Autodesk Inventor part; units mm, degrees
ref_plane "YZ Plane" through (0, 0, 0) normal (1, 0, 0) x (0, 1, 0)
ref_plane "XZ Plane" through (0, 0, 0) normal (0, 1, 0) x (-1, 0, 0)
ref_plane "XY Plane" through (0, 0, 0) normal (0, 0, 1) x (1, 0, 0)
sketch "Sketch1" plane through (0, 0, 0) normal (0, 0, 1) x (1, 0, 0)
  line L0 (-40, 12.5) -> (40, 12.5)
  line L1 (40, 12.5) -> (40, -12.5)
  line L2 (40, -12.5) -> (-40, -12.5)
  line L3 (-40, -12.5) -> (-40, 12.5)
  line L4 (-58.4065, 0) -> (96.114, 0) construction
  line L5 (0, 47.121) -> (0, -49.5625) construction
  line L6 (20, 12.5) -> (20, -12.5)
  line L7 (20, 12.5) -> (40, 5.2206)
  line L8 (20, -12.5) -> (40, -5.2206)
  point P0 (0, 0)
  point P1 (0, 12.5)
  point P2 (40, 0)
  dimension "d0" = 80
  dimension "d1" = 25
  dimension "d11" = 20
  dimension "d16" = 70
  dimension "d17" = 70
extrude "Extrusion4" add sketch "Sketch1" along normal blind 0.2 contours L0 L6 L2 L3 | L7 L1 L8 L6
extrude "Extrusion5" add sketch "Sketch1" along normal blind 0.4 contours L7 L1 L8 L6
equation "\"d18\" = material"
equation "\"d20\" = 2 * material"
properties part number "BandBack"
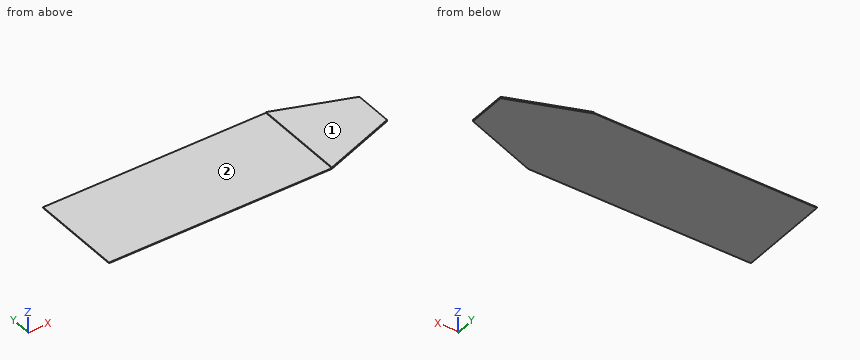
Part model, mm, in its own coordinate system. Face numbers are marked on the shaded views. A direction names the side the tool comes from. Coordinates: 2 decimals unless noted, no trailing zeros. Loops run counter-clockwise (first coordinate to the right, second up) from the corner with the lowest first, then second, coordinate; pieces in that order, holes last. Notation, with made-up numbers: (53, -33.5) -> (79, -33.5) arc R23 cw to (79, -9.5) -> close; hole circle Ø7 at (83, 24). An arc over 180 degrees is marked (long way). Use a Markdown table: item, result. Add a question column.
Item 1: Band-saw the part on A-A on z = 0.1. Write the cut outline in (x, y).
Item 2: Which spindle directions (+Z, -Z, +X, -X, +Y, -Y) get a long thin tool onto all of the face, cutting with end or side? Do the marked faces 1 and 2. Say none if no direction does.
Item 3: Probe probe 1 along Z at (x, y) = (-6, 3.75); probe 2 along Y at (x, z) = (29, 0.3); probe 3 along Y at (x, z) = (30.5, 0.05). List the from-to ranges inside material, lowest first.
Item 4: Band-saw the part on C-C on x = -2. Write the cut outline in (y, z).
Item 5: Band-saw the part on D-D on x = 26.5. Write the cut outline in (y, z).
Item 6: Band-saw the part on B-B on y = 1.75. Write the cut outline in (x, z), plus the area to 3 significant figures.
Item 7: Flat gauge pin, fed straight in: P1, Ø6, axis at x = 8, y = -8, coming from the +Z side. Where does the tip first touch, or does it go through?
Geometry says:
| question | item | result |
|---|---|---|
| 1 | outline | (-40, -12.5) -> (20, -12.5) -> (40, -5.22) -> (40, 5.22) -> (20, 12.5) -> (-40, 12.5) -> close |
| 2 | face 1 | +Z, +X, -X, +Y, -Y |
| 2 | face 2 | +Z, -X, +Y, -Y |
| 3 | probe 1 | 0 to 0.2 |
| 3 | probe 2 | -9.22 to 9.22 |
| 3 | probe 3 | -8.68 to 8.68 |
| 4 | outline | (-12.5, 0) -> (12.5, 0) -> (12.5, 0.2) -> (-12.5, 0.2) -> close |
| 5 | outline | (-10.13, 0) -> (10.13, 0) -> (10.13, 0.4) -> (-10.13, 0.4) -> close |
| 6 | outline | (-40, 0) -> (40, 0) -> (40, 0.4) -> (20, 0.4) -> (20, 0.2) -> (-40, 0.2) -> close |
| 6 | area | 20.0 mm² |
| 7 | P1 | z = 0.2 |
